Verification items for the finished model (mm, model axes). Give positions to 0.01 mm unless a question says otherwise; leave off trailing zeros. Write each loop counter-clockwise with the first axis right and the second up, starting at its lowest first coordinate (ties: lowest second). Pieces come first, ordered by that corner, then holes. Notation, with made-up numbers: (86, -0.75) -> (102, -0.75) arc R27 cw to (102, 16.25) -> close; hole circle Ø9 at (53, 55). An arc over 180 degrees is marked (long way). Answer as CSV lines item,"result". Start each with the question number.
1) Sectioned sample at C-C on y = 49.5. Record the cut outline in (x, z), and give its area (3 significant figures).
2) Gauge pin test, flat ends, axial feed: pin 1 Ø1 at (x, y) = (156, 81) entering from -Z; pin 2 Ø1.5 at (x, y) = (156, 53) entering from +Z; pin 3 Ø0.6 at (y, z) = (-2, -54.5) entering from +X. Record the tip position at first contact, or that the pin passes through.
3) Sectioned sample at A-A on x = 158.8. Record the cut outline in (y, z).
4) Sectioned sample at B-B on z = -130.5. Record the cut outline in (x, y), and give its area (3 significant figures).
5) Material ranges on L1, parallel to Y at x = 159.6, z = -78; L2, parallel to Z at x = 157.95, y = 37.5; L3, parallel to Z at x = 158, y = 75.5, recorded low to high.
6) Sectioned sample at D-D on z = -104.5. Record the cut outline in (x, y).
```python
from build123d import *

# Parameters (mm, degrees)
BOSS_EXTRUDE1_DEPTH = 155
SKETCH4_W           = 144
SKETCH4_H           = 111
CUT_EXTRUDE1_DEPTH  = 5
SKETCH5_R           = 38.5
CUT_EXTRUDE2_DEPTH  = 10
BOSS_EXTRUDE2_DEPTH = 5
CUT_EXTRUDE3_DEPTH  = 5
SKETCH8_W           = 111
SKETCH8_H           = 2
CUT_EXTRUDE4_DEPTH  = 2.5
CUT_EXTRUDE5_DEPTH  = 2.5


with BuildPart() as part:
    # Sketch3 → Boss-Extrude1 (new body)
    with BuildSketch(Plane(origin=(0, 0, 0), x_dir=(0, 0, -1), z_dir=(1, 0, 0))):
        Polygon((58.381197846, 114.119200877), (0.860471904, 14.490381057), (12.979274058, -6.5), (132.75, -6.5), (142.504165125, 10.394709581), (82.618802154, 114.119200877), align=None)
        Polygon((7.5, 12.990381057), (15, 0), (15, -1.5), (126, -1.5), (126, 0), (133.5, 12.990381057), (134.799038106, 13.740381057), (79.299038106, 109.869200877), (78, 109.119200877), (63, 109.119200877), (61.700961894, 109.869200877), (6.200961894, 13.740381057), align=None, mode=Mode.SUBTRACT)
    extrude(amount=BOSS_EXTRUDE1_DEPTH)

    # Sketch4 → Cut-Extrude1 (cut)
    with BuildSketch(Plane(origin=(0, 3.25, 5.629165125), x_dir=(1, 0, 0), z_dir=(0, 0.4999999999999995, 0.8660254037844389))):
        with Locations((77.5, 70.5)):
            Rectangle(SKETCH4_W, SKETCH4_H)
    extrude(amount=-CUT_EXTRUDE1_DEPTH, mode=Mode.SUBTRACT)

    # Sketch5 → Cut-Extrude2 (cut)
    with BuildSketch(Plane(origin=(0, 64.304790967, -111.379165125), x_dir=(-1, 0, 0), z_dir=(0, 0.5000000000000006, -0.8660254037844385))):
        with Locations(Location((-77.5, -2.364637029, 0), (0, 0, 90))):
            Circle(SKETCH5_R)
    extrude(amount=-CUT_EXTRUDE2_DEPTH, mode=Mode.SUBTRACT)


with BuildPart() as body_2:
    # Sketch6 → Boss-Extrude2 (new body)
    with BuildSketch(Plane(origin=(155, 0, 0), x_dir=(0, 0, -1), z_dir=(1, 0, 0))):
        Polygon((82.618802154, 114.119200877), (58.381197846, 114.119200877), (0.860471904, 14.490381057), (12.979274058, -6.5), (132.75, -6.5), (142.504165125, 10.394709581), align=None)
    extrude(amount=BOSS_EXTRUDE2_DEPTH)

    # Sketch7 → Cut-Extrude3 (cut)
    with BuildSketch(Plane(origin=(160, 0, 0), x_dir=(0, 0, -1), z_dir=(1, 0, 0))):
        Polygon((63, 109.119200877), (7.5, 12.990381057), (15, 0), (126, 0), (133.5, 12.990381057), (78, 109.119200877), align=None)
    extrude(amount=-CUT_EXTRUDE3_DEPTH, mode=Mode.SUBTRACT)

    # Sketch8 → Cut-Extrude4 (cut)
    with BuildSketch(Plane(origin=(160, 0, 0), x_dir=(0, 0, -1), z_dir=(1, 0, 0))):
        Polygon((6.200961894, 13.740381057), (61.700961894, 109.869200877), (59.968911087, 110.869200877), (4.468911087, 14.740381057), align=None)
        with Locations((70.5, -2.5)):
            Rectangle(SKETCH8_W, SKETCH8_H)
        Polygon((79.299038106, 109.869200877), (134.799038106, 13.740381057), (136.531088913, 14.740381057), (81.031088913, 110.869200877), align=None)
    extrude(amount=-CUT_EXTRUDE4_DEPTH, mode=Mode.SUBTRACT)

    # Sketch10 → Cut-Extrude5 (cut)
    with BuildSketch(Plane(origin=(160, 0, 0), x_dir=(0, 0, -1), z_dir=(1, 0, 0))):
        Polygon((37.25, 64.518892582), (33.25, 57.590689352), (31.950961894, 58.340689352), (35.950961894, 65.268892582), align=None)
    extrude(amount=-CUT_EXTRUDE5_DEPTH, mode=Mode.SUBTRACT)


solid = body_2.part
```
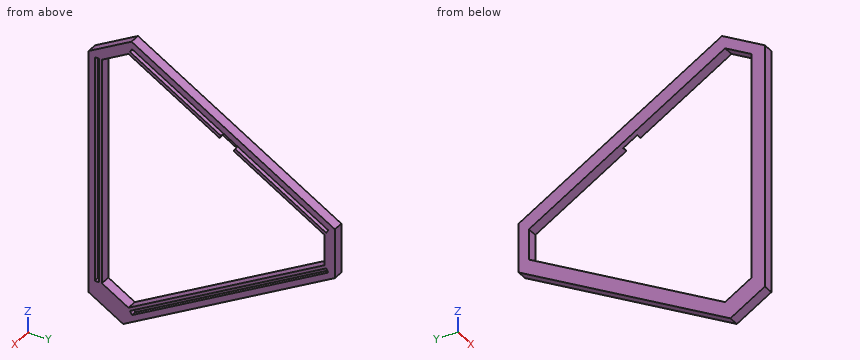
Ans:
1,outline,"(155, -119.93) -> (160, -119.93) -> (160, -116.46) -> (157.5, -116.46) -> (157.5, -114.15) -> (160, -114.15) -> (160, -112.42) -> (155, -112.42) -> close; (155, -28.58) -> (160, -28.58) -> (160, -26.85) -> (157.5, -26.85) -> (157.5, -24.54) -> (160, -24.54) -> (160, -21.07) -> (155, -21.07) -> close"
1,area,"63.5 mm²"
2,pin 1,"stops at z = -102.03"
2,pin 2,"stops at z = -22.66"
2,pin 3,"stops at x = 157.5"
3,outline,"(-6.5, -132.75) -> (10.39, -142.5) -> (114.12, -82.62) -> (114.12, -58.38) -> (14.49, -0.86) -> (-6.5, -12.98) -> close; hole (-3.5, -126) -> (-1.5, -126) -> (-1.5, -15) -> (-3.5, -15) -> close; hole (0, -126) -> (12.99, -133.5) -> (109.12, -78) -> (109.12, -63) -> (64.52, -37.25) -> (65.27, -35.95) -> (109.87, -61.7) -> (110.87, -59.97) -> (14.74, -4.47) -> (13.74, -6.2) -> (58.34, -31.95) -> (57.59, -33.25) -> (12.99, -7.5) -> (0, -15) -> close; hole (13.74, -134.8) -> (14.74, -136.53) -> (110.87, -81.03) -> (109.87, -79.3) -> close"
4,outline,"(155, -6.5) -> (160, -6.5) -> (160, 7.79) -> (155, 7.79) -> close; (155, 18.19) -> (160, 18.19) -> (160, 21.19) -> (157.5, 21.19) -> (157.5, 25.19) -> (160, 25.19) -> (160, 31.19) -> (155, 31.19) -> close"
4,area,"126 mm²"
5,L1,"y = -6.5 to -3.5, -1.5 to 0, 109.12 to 114.12"
5,L2,"z = -126.85 to -123.39, -121.08 to -119.35, -21.65 to -19.92, -17.61 to -14.15"
5,L3,"z = -104.92 to -101.45, -99.14 to -97.41, -43.59 to -41.86, -39.55 to -36.08"
6,outline,"(155, -6.5) -> (160, -6.5) -> (160, -3.5) -> (157.5, -3.5) -> (157.5, -1.5) -> (160, -1.5) -> (160, 0) -> (155, 0) -> close; (155, 63.22) -> (160, 63.22) -> (160, 66.22) -> (157.5, 66.22) -> (157.5, 70.22) -> (160, 70.22) -> (160, 76.22) -> (155, 76.22) -> close"
